```python
from build123d import *

# Parameters (mm, degrees)
SKETCH003_R             = 2
PAD001_DEPTH            = 1.5
SKETCH004_R             = 1
PAD002_DEPTH            = 7
FILLET_R                = 0.2
SKETCH005_W             = 4.5
SKETCH005_H             = 1
POCKET002_DEPTH         = 0.5
BODY001_PLACEMENT_ANGLE = 35


with BuildPart() as part:
    # Sketch003 → Pad001 (new body)
    with BuildSketch(Plane.XY):
        Circle(SKETCH003_R)
    extrude(amount=PAD001_DEPTH)

    # Sketch004 (on Face2 of Pad001) → Pad002 (join)
    with BuildSketch(Plane(origin=(0, 0, 0), x_dir=(1, 0, 0), z_dir=(0, 0, -1))):
        Circle(SKETCH004_R)
    extrude(amount=PAD002_DEPTH)

    # Fillet
    fillet_edges = [part.edges().sort_by_distance(p)[0] for p in [
        (-2, 0, 1.5),
    ]]
    fillet(fillet_edges, radius=FILLET_R)

    # Sketch005 (on Face3 of Pad002) → Pocket002 (cut)
    with BuildSketch(Plane.XY.offset(1.5)):
        Rectangle(SKETCH005_W, SKETCH005_H)
    extrude(amount=-POCKET002_DEPTH, mode=Mode.SUBTRACT)


with BuildPart() as part_1:
    # Body001 placement: moved
    add(part.part.moved(Location((2.54, 0, 16))).rotate(Axis((2.54, 0, 16), (0, 0, 1)), BODY001_PLACEMENT_ANGLE))


solid = part_1.part
```
Read the model definition and answer for the solid it produces. Units are mm, in the model's axes. A direction names the side the tool comes from. Give positions to 0.01 mm unless a question says otherwise; leave off trailing zeros. Write each loop counter-clockwise with the first axis right and the second up, starting at its lowest first coordinate (ties: lowest second). Pieces come first, ordered by that corner, then holes. Notation, with made-up numbers: (49.5, 28.25) -> (93.5, 28.25) arc R26 ccw to (93.5, 56.25) -> close; hole circle Ø10 at (-39, -26.75). An arc over 180 degrees is marked (long way). Answer as a JSON object with one key per item and string values.
1) Flat-ended cylindrical pins translate along their axes: pin 1 Ø2 at (y, z) = (1.5, 11.5) entering from +X; pin 2 Ø1 at (y, z) = (-1, 14.5) entering from -X; pin 3 Ø1.5 at (x, z) = (4, 11) entering from -Y. Find the tip coordinate at first contact, or state that the pin passes through.
Findings below:
{"pin 1": "stops at x = 3.41", "pin 2": "stops at x = 1.67", "pin 3": "stops at y = -0.7"}
2) A tool of negligible diameter and unlimited length cuts with its end or side. For faces 5 (the flat face through (3, 0, 9)), 6 (the flat face through (4, 0, 16)), 7 (the flat face through (3, 0, 17)), from which of +Z, -Z, +X, -X, +Y, -Y can it reach the whole face along a straight path? Write none if from no direction.
Findings below:
{"face 5": "-Z, +X, -X, +Y, -Y", "face 6": "-Z", "face 7": "+Z"}
3) Straight lines are drawn through the part: probe 1 along Z at (x, y) = (2.85, -0.25); probe 2 along Z at (x, y) = (2.6, -1.65); probe 3 along Y at (x, z) = (2.25, 12.75). For each, find the intervals that lie inside material, in ascending order. Write a range as from..to.
Findings below:
{"probe 1": "z = 9..17", "probe 2": "z = 16..17.5", "probe 3": "y = -0.96..0.96"}
4) Section A-A on x = 2.54 is taken. Write down the section's boundary in (y, z).
Findings below:
{"outline": "(-2, 16) -> (-1, 16) -> (-1, 9) -> (1, 9) -> (1, 16) -> (2, 16) -> (2, 17.3) arc R0.2 ccw to (1.8, 17.5) -> (0.61, 17.5) -> (0.61, 17) -> (-0.61, 17) -> (-0.61, 17.5) -> (-1.8, 17.5) arc R0.2 ccw to (-2, 17.3) -> close"}
5) For a pull along X with two mould halves and no side action, classify faces 1 (the cylindrical face through (4.5, 0.4, 16.6)), 2 (the flat face through (2.231, 0.394, 17.254)), 3 (the flat face through (2.8, -0.43, 17.25)), 4 (the flat face through (3, -1, 17.5)) as pulls with the +X half, pulls with the -X half, needs draft (parallel to the pull), parting line crosses it, or undercut.
Findings below:
{"face 1": "parting line crosses it", "face 2": "undercut", "face 3": "undercut", "face 4": "needs draft"}
6) Section C-C on z = 15 is taken. Write down the section's boundary in (x, y), then the cut area to 3 significant figures.
Findings below:
{"outline": "circle Ø2 at (2.54, 0)", "area": "3.14 mm^2"}
7) Section B-B on y = 0 is taken. Write down the section's boundary in (x, z), then the cut area to 3 significant figures.
Findings below:
{"outline": "(0.54, 16) -> (1.54, 16) -> (1.54, 9) -> (3.54, 9) -> (3.54, 16) -> (4.54, 16) -> (4.54, 17.3) arc R0.2 ccw to (4.34, 17.5) -> (3.41, 17.5) -> (3.41, 17) -> (1.67, 17) -> (1.67, 17.5) -> (0.74, 17.5) arc R0.2 ccw to (0.54, 17.3) -> close", "area": "19.1 mm^2"}
